For this review, take the finished solid that the model builds, in its own axes (mm). Round coordinates to 2 decimals unless told otherwise and drop trailing zeros. Order: outer loops, then holes, each group sorted by start corner. A loop starts at its lowest first (then second) coordinate and runs counter-clockwise, first axis right, second up. Notation, with made-up numbers: M 36.5,44 L 65.5,44 A10 cw 65.5,48 Z; hole C 50.25,62.5 d1. An arc over 180 degrees is marked long. Answer as a JSON object with one key per item and string values.
Autodesk Inventor part; units mm, degrees
ref_plane "YZ Plane" through (0, 0, 0) normal (1, 0, 0) x (0, 1, 0)
ref_plane "XZ Plane" through (0, 0, 0) normal (0, 1, 0) x (-1, 0, 0)
ref_plane "XY Plane" through (0, 0, 0) normal (0, 0, 1) x (1, 0, 0)
sketch "Sketch1" plane through (0, 0, 0) normal (0, 0, 1) x (1, 0, 0)
  line L0 (800, 0) -> (800, -485) construction
  line L1 (800, -485) -> (0, -485)
  line L2 (800, 0) -> (777.7845, -423.8974)
  line L3 (735, -485) -> (800, -392.1704)
  line L4 (0, -485) -> (0, 0)
  line L5 (0, 0) -> (800, 0)
  dimension "d9" = 800
  dimension "d10" = 35
  dimension "d11" = 485
  dimension "d12" = 3
  dimension "d13" = 65
extrude "Plate1" add sketch "Sketch1" along normal blind 2
mirror "Mirror1" about plane through (0, 0, 0) normal (1, 0, 0)
sketch "Sketch2" plane through (0, 0, 2) normal (0, 0, 1) x (1, 0, 0)
  line L0 (-55, -435) -> (-55, -423) construction
  line L1 (-55, -423) -> (55, -423) construction
  line L2 (55, -423) -> (55, -435) construction
  line L3 (55, -435) -> (-55, -435) construction
  line L4 (-735, -485) -> (735, -485)
  point P0 (0, 0)
  point P1 (0, -435)
  point P2 (0, -485)
  dimension "d6" = 12
  dimension "d7" = 110
  dimension "d8" = 50
mark "Mark1"
equation "\"d2\" = Thickness"
equation "\"BendReliefWidth\" = Thickness"
equation "\"BendReliefDepth\" = 0.5 * Thickness"
equation "\"CornerReliefSize\" = 4 * Thickness"
equation "\"MinimumRemnant\" = 2 * Thickness"
equation "\"TransitionRadius\" = BendRadius"
equation "\"JacobiRadiusSize\" = BendRadius"
equation "\"GapSize\" = Thickness"
properties part number "MSC 703 FACE 3" material "AISI304"
1) Add section A-A on z = 1.35. State the section outline as (x, y) points.
Geometry check:
{"outline": "M -800,0 L -777.78,-423.9 L -735,-485 L 735,-485 L 777.78,-423.9 L 800,0 Z"}
2) For L1, parallel to X at y = -377.5, z = 0.8; L2, parallel to X at y = -345.5, z = 0.2, list the stretches that pass through material, from the lowest coordinate up.
Geometry check:
{"L1": "x = -780.22 to 780.22", "L2": "x = -781.89 to 781.89"}
3) Add section B-B on y = -374. State the section outline as (x, z) points, and give its area (3 significant figures).
Geometry check:
{"outline": "M -780.4,0 L 780.4,0 L 780.4,2 L -780.4,2 Z", "area": "3,120 mm²"}
4) Add section C-C on y = -276. State the section outline as (x, z) points.
Geometry check:
{"outline": "M -785.54,0 L 785.54,0 L 785.54,2 L -785.54,2 Z"}
